Model file for the job. Use its own axes, mm. Face numbers are marked on the shaded views. A direction names the side the tool comes from. Round coordinates to 2 decimals unless told otherwise and drop trailing zeros. Loops run counter-clockwise (first coordinate to the right, second up) from the corner with the lowest first, then second, coordinate; pieces in that order, holes last. Notation, with made-up numbers: (-5, 33.5) - (0, 33.5) arc R19 cw to (0, 60.5) - close; hole circle Ø1 at (54.5, 80.25). An arc over 180 degrees is marked (long way). Use one line per item in the form item = value.
from build123d import *
from build123d.topology import SkipClean

# Parameters (mm, degrees)
BOSS_EXTRUDE1_DEPTH = 5
SKETCH7_W           = 17.76
SKETCH7_H           = 7.76
BOSS_EXTRUDE2_DEPTH = 23
SKETCH8_R           = 1.25
CUT_EXTRUDE1_DEPTH  = 5
CUT_EXTRUDE2_START  = -5
SKETCH9_R           = 1.25
CUT_EXTRUDE2_DEPTH  = 5
BOSS_EXTRUDE3_DEPTH = 25
FILLET1_R           = 22
FILLET2_R           = 30


with BuildPart() as part:
    # Sketch5 → Boss-Extrude1 (new body)
    with BuildSketch(Plane(origin=(0, 0, 0), x_dir=(1, 0, 0), z_dir=(0, 1, 0))):
        with BuildLine():
            Line((-7.71, 88.14), (-7.71, -30))
            Line((-7.71, -30), (-2.06, -30))
            Line((-2.06, -30), (-2.06, -14.77))
            ThreePointArc((-2.06, -14.77), (-4.31, -12.52), (-2.06, -10.27))
            Line((-2.06, -10.27), (-2.06, 93.1))
            ThreePointArc((-2.06, 93.1), (-4.31, 95.35), (-2.06, 97.6))
            Line((-2.06, 97.6), (-2.06, 105.16))
            Line((-2.06, 105.16), (-74.3, 105.16))
            Line((-74.3, 105.16), (-74.3, 146.76))
            Line((-74.3, 146.76), (-109.82, 146.76))
            Line((-109.82, 146.76), (-109.82, 88.14))
            Line((-109.82, 88.14), (-7.71, 88.14))
        make_face()
    boss_extrude1 = extrude(amount=BOSS_EXTRUDE1_DEPTH)

    # Sketch7 → Boss-Extrude2 (add)
    with BuildSketch(Plane(origin=(0, 5, 0), x_dir=(1, 0, 0), z_dir=(0, 1, 0))):
        Polygon((-109.82, 146.76), (-109.82, 88.14), (-74.3, 88.14), (-74.3, 95.9), (-102.06, 95.9), (-102.06, 146.76), align=None)
        with Locations((-83.18, 142.88)):
            Rectangle(SKETCH7_W, SKETCH7_H)
    boss_extrude2 = extrude(amount=BOSS_EXTRUDE2_DEPTH)

    # Sketch8 → Cut-Extrude1 (cut)
    with BuildSketch(Plane(origin=(-74.3, 0, 0), x_dir=(0, 0, -1), z_dir=(1, 0, 0))):
        with Locations((92.02, 10)):
            Circle(SKETCH8_R)
        with Locations((92.02, 20)):
            Circle(SKETCH8_R)
        with Locations((142.88, 10)):
            Circle(SKETCH8_R)
        with Locations((142.88, 20)):
            Circle(SKETCH8_R)
    extrude(amount=-CUT_EXTRUDE1_DEPTH, mode=Mode.SUBTRACT)

    # Mirror2: Boss-Extrude1, Boss-Extrude2 across plane
    with SkipClean():  # the faces are left unmerged after this step: merging them gives an invalid solid
        add(boss_extrude1.mirror(Plane(origin=(-2.06, 5, 0), x_dir=(0, 0, 1), z_dir=(1, 0, 0))))
        add(boss_extrude2.mirror(Plane(origin=(-2.06, 5, 0), x_dir=(0, 0, 1), z_dir=(1, 0, 0))))

    # Sketch9 → Cut-Extrude2 (cut)
    with SkipClean():  # the faces are left unmerged after this step: merging them gives an invalid solid
        with BuildSketch(Plane.ZY.offset(-70.18).offset(CUT_EXTRUDE2_START)):
            with Locations(Location((-142.88, 10, 0), (0, 0, 180))):
                Circle(SKETCH9_R)
            with Locations(Location((-142.88, 20, 0), (0, 0, 180))):
                Circle(SKETCH9_R)
            with Locations(Location((-92.02, 10, 0), (0, 0, 180))):
                Circle(SKETCH9_R)
            with Locations(Location((-92.02, 20, 0), (0, 0, 180))):
                Circle(SKETCH9_R)
        extrude(amount=CUT_EXTRUDE2_DEPTH, mode=Mode.SUBTRACT)

    # Sketch12 → Boss-Extrude3 (add)
    with SkipClean():  # the faces are left unmerged after this step: merging them gives an invalid solid
        with BuildSketch(Plane(origin=(-60.728648392, 0, 0), x_dir=(0, 0, -1), z_dir=(1, 0, 0))):
            with BuildLine():
                Line((130.792872119, -14.205030824), (130.268072642, -10.239607075))
                ThreePointArc((130.268072642, -10.239607075), (114.312520733, -7.123943435), (103.482147137, 5))
                Line((103.482147137, 5), (99.183531943, 5))
                ThreePointArc((99.183531943, 5), (111.604669447, -10.171432922), (130.792872119, -14.205030824))
            make_face()
        boss_extrude3 = extrude(amount=BOSS_EXTRUDE3_DEPTH)

    # Mirror3: Boss-Extrude3 across plane
    with SkipClean():  # the faces are left unmerged after this step: merging them gives an invalid solid
        add(boss_extrude3.mirror(Plane(origin=(-2.06, 0, 0), x_dir=(0, 0, 1), z_dir=(1, 0, 0))))

    # Fillet1
    # the kernel refuses this fillet: 22 mm, written as the material it adds along each edge
    with BuildSketch(Plane(origin=(-35.728648392, 1.749196605, -105.16), x_dir=(0, 1, 0), z_dir=(-1, 0, 0))) as fillet1_piece_1:
        with BuildLine():
            CenterArc((9.879940472, 20.977477008), FILLET1_R, 192.960861786, 59.501970429)
            Line((-11.559576515, 16.043197795), (-11.988366855, 15.94451221))
            ThreePointArc((-11.988366855, 15.94451221), (-7.755155531, 6.598291061), (-0.22933098, -0.375509389))
            Line((-0.22933098, -0.375509389), (0, -0.44))
            ThreePointArc((0, -0.44), (1.625401698, -0.44), (3.118220654, -0.41954954))
            Line((3.118220654, -0.41954954), (3.250803395, 0))
        make_face()
    extrude(amount=25)
    with BuildSketch(Plane(origin=(31.608648392, 1.749196605, -105.16), x_dir=(0, 1, 0), z_dir=(1, 0, 0))) as fillet1_piece_2:
        with BuildLine():
            CenterArc((9.879940472, -20.977477008), FILLET1_R, 107.537167785, 59.501970429)
            Line((-11.559576515, -16.043197795), (-11.988366855, -15.94451221))
            ThreePointArc((-11.988366855, -15.94451221), (-7.755155531, -6.598291061), (-0.22933098, 0.375509389))
            Line((-0.22933098, 0.375509389), (0, 0.44))
            ThreePointArc((0, 0.44), (1.625401698, 0.44), (3.118220654, 0.41954954))
            Line((3.118220654, 0.41954954), (3.250803395, 0))
        make_face()
    extrude(amount=25)

    # Fillet2
    # the kernel refuses this fillet: 30 mm, written as the material it adds along each edge
    with BuildSketch(Plane(origin=(-1.974069594, 0, -101.544349118), x_dir=(0, 0, 1), z_dir=(-1, 0, 0))) as fillet2_piece_1_section:
        with BuildLine():
            CenterArc((13.501831519, -30), FILLET2_R, 90, 40.801822192)
            ThreePointArc((-6.101508838, -7.290771769), (-2.755120907, -3.892795973), (0, 0))
            Line((0, 0), (13.501831519, 0))
        make_face()
    fillet2_piece_1 = extrude(amount=58.754578797, mode=Mode.PRIVATE)
    fillet2_piece_1 = split(fillet2_piece_1, bisect_by=Plane(origin=(-4.842034797, 0.299973601, -88.14), z_dir=(0, 0, 1)), keep=Keep.TOP, mode=Mode.PRIVATE)
    fillet2_piece_1 = split(fillet2_piece_1, bisect_by=Plane(origin=(-7.71, 0.299973601, -88.091260944), z_dir=(1, 0, 0)), keep=Keep.TOP, mode=Mode.PRIVATE)
    add(fillet2_piece_1)
    with BuildSketch(Plane(origin=(-35.728648392, 0, -101.544349118), x_dir=(0, 0, 1), z_dir=(-1, 0, 0))) as fillet2_piece_2_section:
        with BuildLine():
            CenterArc((13.501831519, -30), FILLET2_R, 90, 40.801822192)
            ThreePointArc((-6.101508838, -7.290771769), (-2.755120907, -3.892795973), (0, 0))
            Line((0, 0), (13.501831519, 0))
        make_face()
    fillet2_piece_2 = extrude(amount=25, mode=Mode.PRIVATE)
    fillet2_piece_2 = split(fillet2_piece_2, bisect_by=Plane(origin=(-48.228648392, -1.487894786, -88.14), z_dir=(0, 0, -1)), keep=Keep.TOP, mode=Mode.PRIVATE)
    add(fillet2_piece_2)
    with BuildSketch(Plane(origin=(-2.145930406, 0, -101.544349118), x_dir=(0, 0, 1), z_dir=(1, 0, 0))) as fillet2_piece_3_section:
        with BuildLine():
            CenterArc((13.501831519, 30), FILLET2_R, 229.198177808, 40.801822192)
            ThreePointArc((-6.101508838, 7.290771769), (-2.755120907, 3.892795973), (0, 0))
            Line((0, 0), (13.501831519, 0))
        make_face()
    fillet2_piece_3 = extrude(amount=58.754578797, mode=Mode.PRIVATE)
    fillet2_piece_3 = split(fillet2_piece_3, bisect_by=Plane(origin=(3.59, 0.299973601, -88.091260944), z_dir=(-1, 0, 0)), keep=Keep.TOP, mode=Mode.PRIVATE)
    fillet2_piece_3 = split(fillet2_piece_3, bisect_by=Plane(origin=(0.722034797, 0.299973601, -88.14), z_dir=(0, 0, 1)), keep=Keep.TOP, mode=Mode.PRIVATE)
    add(fillet2_piece_3)
    with BuildSketch(Plane(origin=(31.608648392, 0, -101.544349118), x_dir=(0, 0, 1), z_dir=(1, 0, 0))) as fillet2_piece_4_section:
        with BuildLine():
            CenterArc((13.501831519, 30), FILLET2_R, 229.198177808, 40.801822192)
            ThreePointArc((-6.101508838, 7.290771769), (-2.755120907, 3.892795973), (0, 0))
            Line((0, 0), (13.501831519, 0))
        make_face()
    fillet2_piece_4 = extrude(amount=25, mode=Mode.PRIVATE)
    fillet2_piece_4 = split(fillet2_piece_4, bisect_by=Plane(origin=(44.108648392, -1.487894786, -88.14), z_dir=(0, 0, -1)), keep=Keep.TOP, mode=Mode.PRIVATE)
    add(fillet2_piece_4)


solid = part.part
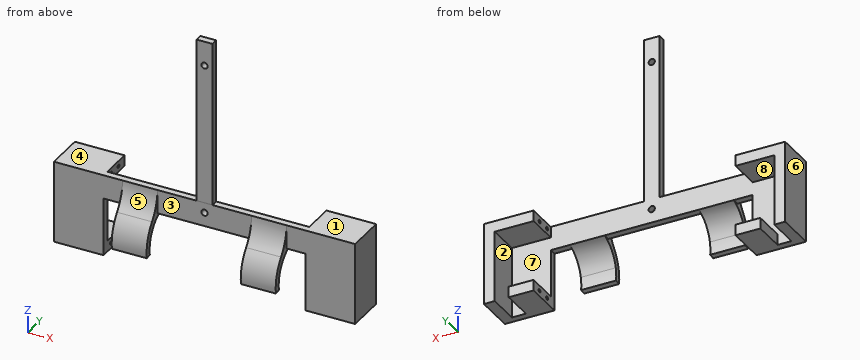
1. Cut at A-A, the plane y = 25. Give the cut face in (x, z).
Geometry check:
outline = (-109.82, -146.76) - (-102.06, -146.76) - (-102.06, -95.9) - (-74.3, -95.9) - (-74.3, -88.14) - (-109.82, -88.14) - close; (-92.06, -146.76) - (-74.3, -146.76) - (-74.3, -139) - (-92.06, -139) - close; (70.18, -146.76) - (87.94, -146.76) - (87.94, -139) - (70.18, -139) - close; (70.18, -95.9) - (97.94, -95.9) - (97.94, -146.76) - (105.7, -146.76) - (105.7, -88.14) - (70.18, -88.14) - close
2. Wall check: probe 1 along Y at (x, z) = (-75.25, -142.88); probe 2 along X at (y, z) = (17.5, -110); probe 3 along Z at (x, y) = (-80.5, 7). Give the ranges that are in metal, low to high.
Geometry check:
probe_1 = 0 to 8.75, 11.25 to 18.75, 21.25 to 28
probe_2 = -109.82 to -102.06, 97.94 to 105.7
probe_3 = -146.76 to -139, -95.9 to -88.14
3. Cut at D-D, the plane x = 62.5. Give the cut face in (y, z).
Geometry check:
outline = (0, -105.16) - (5, -105.16) - (5, -88.14) - (0, -88.14) - close
4. Pull direction X, two halves, no side cores. Call the marked faces 5, 6, 7 and 8: +X half, -X half, draft (parallel to the pull), parting line (faces both ways), or undercut.
Geometry check:
face_5 = draft
face_6 = -X half
face_7 = undercut
face_8 = undercut
5. Flat gauge pins, fed straight in: pin 1 (5 mm diameter, centred on x = -44.5, z = -113, fed in from -Y); pin 2 (1.5 mm diameter, centred on x = -14, y = 2.5, fed in from -Z); pin 3 (6 mm diameter, centred on y = -7.5, z = -127.5, fed in from -X). Where does each tip first touch, or does it go through?
Geometry check:
pin_1 = -12.16
pin_2 = -105.16
pin_3 = -60.73
6. Tool access for the marked faces 1, 2, 3 and 4: list every direction of +Z, -Z, +X, -X, +Y, -Y with a clear straight run to the whole face (end or side of a thin tool).
Geometry check:
face_1 = +Z, +X, +Y, -Y
face_2 = -Z, +Y
face_3 = +Z, -Z, -Y
face_4 = +Z, -X, +Y, -Y
7. Cut at C-C, the plane z = -52.5. Give the cut face in (x, y).
Geometry check:
outline = (-7.71, 0) - (3.59, 0) - (3.59, 5) - (-7.71, 5) - close
8. Cut at B-B, the plane z = -125.5. Give the cut face in (x, y).
Geometry check:
outline = (-109.82, 0) - (-74.3, 0) - (-74.3, 5) - (-102.06, 5) - (-102.06, 28) - (-109.82, 28) - close; (-60.73, -14.43) - (-35.73, -14.43) - (-35.73, -10.42) - (-60.73, -10.42) - close; (31.61, -14.43) - (56.61, -14.43) - (56.61, -10.42) - (31.61, -10.42) - close; (70.18, 0) - (105.7, 0) - (105.7, 28) - (97.94, 28) - (97.94, 5) - (70.18, 5) - close
